Geometry: final body of the model. Coordinates: model frame, mm. A direction names the side the tool comes from. Give positions to 0.01 mm unless a question says otherwise; leave off trailing zeros. Loops run counter-clockwise (first coordinate to the right, second up) from the corner with the lowest first, then second, coordinate; pieces in that order, holes last. Notation, with made-up numbers: (-37.5, -28.5) -> (-6.5, -28.5) arc R27 cw to (-6.5, -1.5) -> close; hole circle Ø2 at (86.5, 89). An arc over 180 degrees is marked (long way). One line per item, written item: value. Start each with the question number.
from build123d import *

# Parameters (mm, degrees)
F0_W     = 228.6
F0_H     = 101.6
F1_DEPTH = 19.05


with BuildPart() as f1:
    # F0 (on Right) → F1 (new body)
    with BuildSketch(Plane.YZ):
        Polygon((-114.3, -241.3), (-114.3, 342.9), (-228.6, 342.9), (-228.6, -342.9), (-114.3, -342.9), align=None)
        with Locations((0, -292.1)):
            Rectangle(F0_W, F0_H)
        Polygon((228.6, -342.9), (228.6, 342.9), (114.3, 342.9), (114.3, -241.3), (114.3, -342.9), align=None)
    extrude(amount=F1_DEPTH)


solid = f1.part
Item 1: Ray query, line 1 along Y through (x, z) = (14.5, -25); line 2 along Z through (x, y) = (16.75, 108). Return the intervals inside material, ascending. Write a range as [from, to].
Item 2: Section B-B, the plane x = 5. Output: boundary loops of the cut face in (y, z), then the cut area to 3 significant figures.
Item 3: Section A-A, the plane z = -15. Output: boundary loops of the cut face in (x, y), then the cut area to 3 significant figures.
Item 4: Mould query, pull axis Y, two halves, no side actions, for faces 1 (the face through (0, -156, 5)), 2 (the face through (9, 114.3, 55)), 3 (the face through (9, -228.6, 5)). Classes: pulls with the +Y half, pulls with the -Y half, needs draft (parallel to the pull), parting line crosses it, or undercut.
Item 5: Pin query (flat end, axial travel): pin 1 (5 mm diameter, centred on x = 6, y = -46.5, fed in from +Z). Return the tip coordinate at first contact, or that it passes through.
Item 6: Section C-C, the plane y = -8. Output: boundary loops of the cut face in (x, z).
Item 7: Access query for faces 4 (the face through (9, 172, 342.9)), 5 (the face through (9, -2, -241.3)). Directions: +Z, -Z, +X, -X, +Y, -Y. A direction counts if a zero-diameter tool reaches every point of the face in a straight line with its end or side. Return the directions, or none.
Geometry check:
1. line 1: y = [-228.6, -114.3], [114.3, 228.6]
1. line 2: z = [-342.9, -241.3]
2. outline: (-228.6, -342.9) -> (228.6, -342.9) -> (228.6, 342.9) -> (114.3, 342.9) -> (114.3, -241.3) -> (-114.3, -241.3) -> (-114.3, 342.9) -> (-228.6, 342.9) -> close
2. area: 180,000 mm2
3. outline: (0, -228.6) -> (19.05, -228.6) -> (19.05, -114.3) -> (0, -114.3) -> close; (0, 114.3) -> (19.05, 114.3) -> (19.05, 228.6) -> (0, 228.6) -> close
3. area: 4,350 mm2
4. face 1: needs draft
4. face 2: undercut
4. face 3: pulls with the -Y half
5. pin 1: stops at z = -241.3
6. outline: (0, -342.9) -> (19.05, -342.9) -> (19.05, -241.3) -> (0, -241.3) -> close
7. face 4: +Z, +X, -X, +Y, -Y
7. face 5: +Z, +X, -X
